Design review of the part built by this model. Coordinates are the model's own, in mm. A direction names the side the tool comes from. Coordinates: 2 decimals unless noted, no trailing zeros. Loops run counter-clockwise (first coordinate to the right, second up) from the corner with the lowest first, then second, coordinate; pieces in that order, holes last. Notation, with made-up numbers: (39.5, -35) - (43.5, -35) arc R19 cw to (43.5, 0) - close; hole circle Ø5 at (-9, -31). An arc over 180 degrees is marked (long way). Return JSON: item names as keys, results as strings. Group by question number.
from build123d import *

# Parameters (mm, degrees)
F1_DEPTH    = 19.05
F2_T1_DEPTH = 36.0210888614


# Not quite as in the source:
# - a fillet or chamfer that OpenCascade refuses, or shapes differently, is made with other operations: its cross-section is extruded or revolved along the edge and cut away or added


with BuildPart() as f1:
    # F0 (on Front) → F1 (new body)
    with BuildSketch(Plane.XZ):
        with BuildLine():
            ThreePointArc((8.4433957221, 9.4867838955), (11.5870860373, 5.1989842435), (12.7, 0))
            ThreePointArc((12.7, 0), (-4.5170700973, -11.869544125), (-9.4867838955, 8.4433957221))
            Line((-9.4867838955, 8.4433957221), (-11.3841406746, 10.1320748666))
            ThreePointArc((-11.3841406746, 10.1320748666), (-5.4204841167, -14.24345295), (15.24, 0))
            ThreePointArc((15.24, 0), (13.9045032448, 6.2387810922), (10.1320748666, 11.3841406746))
            Line((10.1320748666, 11.3841406746), (8.4433957221, 9.4867838955))
        make_face()
    extrude(amount=F1_DEPTH)

    # F2: fillet of radius 5.08 on 2 edges, made by hand

    # F2_s2 → F2_t1 (cut)
    with BuildSketch(Plane.XZ.offset(-8.4855444307)):
        with BuildLine():
            ThreePointArc((-11.3843237056, 5.6291361473), (-10.8580531921, 7.8805841193), (-11.3841406746, 10.1320748666))
            Line((-11.3841406746, 10.1320748666), (-9.4867838955, 8.4433957221))
            ThreePointArc((-9.4867838955, 8.4433957221), (-10.5299951264, 7.0999438475), (-11.3843237056, 5.6291361473))
        make_face()
        with BuildLine():
            ThreePointArc((10.6545556025, 6.9116166642), (9.8706902669, 9.0868255644), (10.1320748666, 11.3841406746))
            Line((10.1320748666, 11.3841406746), (8.4433957221, 9.4867838955))
            ThreePointArc((8.4433957221, 9.4867838955), (9.6353934931, 8.2734026998), (10.6545556025, 6.9116166642))
        make_face()
    extrude(amount=F2_T1_DEPTH, mode=Mode.SUBTRACT)


solid = f1.part
Item 1: Add section D-D (x = -4.5). State the section outline as (y, z) points.
Item 2: To check wall thickness, follow line 1 (X direction, y = -14, z = 0); line 2 (Z direction, x = 0, y = -12); line 3 (X direction, y = -8.75, z = 6.75). State the ranges of each line that lie inside material, in increasing order. Write a range as from..to.
Item 3: Add section A-A (z = 8). State the section outline as (x, y) points.
Item 4: Add section C-C (y = -12.75). State the section outline as (x, z) points.
Item 5: For faces 1 (the face through (2, -19.05, -13)), 2 (the face through (9.875, -9.392, 9.054)), list the 3-axis set-ups (+Z, -Z, +X, -X, +Y, -Y) from which the entire face can be reached by the end or side of a thin tool; tool diameter is ignored.
Item 6: Draft analysis for pull direction Z (two halves, no side actions). For faces 3 (the face through (-10.86, -9.39, 7.85)), 4 (the face through (2, 0, -13)), state which applies: pulls with the +Z half, pulls with the -Z half, needs draft (parallel to the pull), parting line crosses it, or undercut.
Item 7: For P1, Ø5, axis at x = 2.5, y = -13, coming from the +Z side; P2, Ø1.5, axis at y = -9, z = 3, coming from the -X side; P3, Ø4, axis at y = -13.5, z = -9.5, coming from the +X side, all flat-tipped, find the tip position at first contact; note any pin that passes through.
Item 8: Add section B-B (x = 12). State the section outline as (y, z) points, then the cut area to 3 significant figures.
Answers below:
{
 "1": {"outline": "(-19.05, -14.56) - (0, -14.56) - (0, -11.88) - (-19.05, -11.88) - close"},
 "2": {"line 1": "x = -15.24..-12.7, 12.7..15.24", "line 2": "z = -15.24..-12.7", "line 3": "x = -13.66..-10.99, 10.76..13.66"},
 "3": {"outline": "(-12.97, -19.05) - (-10.86, -19.05) - (-10.86, 0) - (-12.97, 0) - close; (10.12, -19.05) - (12.97, -19.05) - (12.97, 0) - (10.12, 0) - close"},
 "4": {"outline": "(-11.38, 5.63) arc R5.08 ccw to (-11.38, 10.13) arc R15.24 ccw (long way) to (10.13, 11.38) arc R5.08 ccw to (10.65, 6.91) arc R12.7 cw (long way) to start"},
 "5": {"face 1": "+Z, -Z, +X, -X, -Y", "face 2": "+Y, -Y"},
 "6": {"face 3": "undercut", "face 4": "needs draft"},
 "7": {"P1": "stops at z = -11.67", "P2": "stops at x = -15.07", "P3": "stops at x = 13.27"},
 "8": {"outline": "(-19.05, -9.39) - (0, -9.39) - (0, -4.16) - (-19.05, -4.16) - close; (-19.05, 4.16) - (0, 4.16) - (0, 9.39) - (-19.05, 9.39) - close", "area": "200 mm^2"}
}
